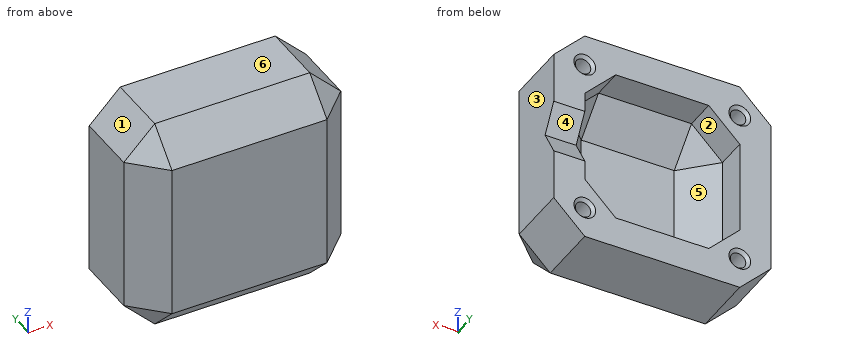
Autodesk Inventor part; units mm, degrees
ref_plane "YZ Plane" through (0, 0, 0) normal (1, 0, 0) x (0, 1, 0)
ref_plane "XZ Plane" through (0, 0, 0) normal (0, 1, 0) x (-1, 0, 0)
ref_plane "XY Plane" through (0, 0, 0) normal (0, 0, 1) x (1, 0, 0)
sketch "Sketch2" plane through (0, 0, 0) normal (0, 1, 0) x (-1, 0, 0)
  line L0 (25, -25) -> (-25, -25)
  line L1 (-25, -25) -> (-25, 25)
  line L2 (-25, 25) -> (25, 25)
  line L3 (25, 25) -> (25, -25)
  line L4 (25, -25) -> (-25, 25) construction
  line L5 (-25, -25) -> (25, 25) construction
  line L6 (35, 35) -> (-35, 35)
  line L7 (-35, 35) -> (-35, -35)
  line L8 (-35, -35) -> (35, -35)
  line L9 (35, -35) -> (35, 35)
  point P0 (0, 0)
  dimension "d0" = 50
  dimension "d1" = 10
  dimension "d19" = 50
extrude "Extrusion1" add sketch "Sketch2" along normal mid plane 30
sketch "Sketch3" plane through (0, -15, 0) normal (0, -1, 0) x (1, 0, 0)
  line L0 (35, -35) -> (35, 35)
  line L1 (35, 35) -> (-35, 35)
  line L2 (-35, 35) -> (-35, -35)
  line L3 (-35, -35) -> (35, -35)
  point P0 (0, 0)
extrude "Extrusion2" add sketch "Sketch3" against normal blind 10
chamfer "Chamfer1" distance 10 angle 45 16 edges at (35, 0, 35) (25, 5, 25) (-25, 5, 25) (-35, 0, 35) (-25, 5, -25) (25, 5, -25) (-35, 0, -35) (35, 0, -35) (0, -5, -25) (25, -5, 0) (0, -5, 25) (-25, -5, 0) (0, -15, -35) (35, -15, 0) (0, -15, 35) (-35, -15, 0)
sketch "Sketch4" plane through (35, -5, -25) normal (1, 0, 0) x (0, 0, -1)
  line L0 (0, 20) -> (0, 0) construction
  line L1 (-50, 20) -> (0, 20) construction
  line L2 (-16.3397, 30) -> (-16.3397, 20)
  line L3 (-16.3397, 20) -> (-25, 15)
  line L4 (-25, 15) -> (-33.6603, 20)
  line L5 (-33.6603, 20) -> (-33.6603, 30)
  line L6 (-33.6603, 30) -> (-25, 35)
  line L7 (-25, 35) -> (-16.3397, 30)
  point P0 (-25, 5)
  point P1 (-25, 25)
  dimension "d9" = 10
  dimension "d10" = 5
  dimension "d20" = 0
extrude "Extrusion3" cut sketch "Sketch4" against normal blind 10
sketch "Sketch5" plane through (0, 15, 0) normal (0, 1, 0) x (1, 0, 0)
  line L0 (-25, 25) -> (-25, 35) construction
  circle A0 centre (-25, 25) radius 2.5
  line L1 (25, 25) -> (35, 25) construction
  circle A1 centre (25, 25) radius 2.5
  line L2 (-25, -25) -> (-35, -25) construction
  circle A2 centre (-25, -25) radius 2.5
  line L3 (-25, -25) -> (25, -25) construction
  circle A3 centre (25, -25) radius 2.5
  point P0 (0, 0)
  dimension "d13" = 5
  dimension "d14" = 5
  dimension "d15" = 5
  dimension "d16" = 5
extrude "Extrusion4" cut sketch "Sketch5" against normal blind 10
chamfer "Chamfer2" distance 1 angle 45 4 edges at (-27.5, 15, 25) (-27.5, 15, -25) (22.5, 15, 25) (22.5, 15, -25)
properties part number "pokemon_ball_white"
Build history of the part. All positions in model axes, mm. Face numbers are marked on the shaded views. A direction names the side the tool comes from. Round coordinates to 2 decimals unless told otherwise and drop trailing zeros. Write each loop counter-clockwise with the first axis right and the second up, starting at its lowest first coordinate (ties: lowest second). Pieces come first, ordered by that corner, then holes. Notation, with made-up numbers: M 82,55.25 L 120,55.25 A16 ccw 120,67.25 Z; hole C 45.5,55.25 d8. An arc over 180 degrees is marked long. Answer as a JSON object with one key per item and string values. Group by question number.
(1) Which spindle directions (+Z, -Z, +X, -X, +Y, -Y) get a long thin tool onto all of the face, cutting with end or side? Do the marked faces 4, 5 and 6. Say none if no direction does.
(2) Drill centre lines: L1, parallel to Z at x = -8, y = 9; L2, parallel to Y at x = 10.5, z = -2; L3, parallel to X at y = 3.5, z = 31.5. Where is each one in solid material? Low to high.
(3) Cut at B-B (x = 19). Give the cut face in (y, z), and give its area (3 significant figures).
(4) Cut at D-D (z = -11). Give the cut face in (x, y), and give its area (3 significant figures).
(5) Mould opens along X. For the marked faces 1, 2 and 3 say: pulls with the +X half, pulls with the -X half, needs draft (parallel to the pull), parting line crosses it, or undercut.
(6) Cut at C-C (y = 8). Give the cut face in (x, z), and give its area (3 significant figures).
(7) Flat gauge pins, fed straight in: pin 1 (5.5 mm diameter, centred on x = 25, z = 25.5, fed in from +Y); pin 2 (4 mm diameter, centred on x = 24, z = -26, fed in from +Y); pin 3 (3 mm diameter, centred on x = 25, z = -25, fed in from +Y); pin 4 (5.5 mm diameter, centred on x = -26, z = 25.5, fed in from +Y). Where does each tip first touch, or does it go through?
(8) Cut at A-A (y = -4). Give the cut face in (x, z), and give its area (3 significant figures).
Responses:
{
 "1": {"face 4": "+X, +Y", "face 5": "+Y", "face 6": "+Z, +X, -X, +Y, -Y"},
 "2": {"L1": "z = -35 to -25, 25 to 35", "L2": "y = -15 to -5", "L3": "x = -28.5 to 28.5"},
 "3": {"outline": "M -15,-25 L -5,-35 L 15,-35 L 15,-21 L 5,-21 L -1,-15 L -1,15 L 5,21 L 15,21 L 15,35 L -5,35 L -15,25 Z", "area": "1,360 mm2"},
 "4": {"outline": "M -35,-5 L -25,-15 L 25,-15 L 35,-5 L 35,15 L 25,15 L 25,5 L 15,-5 L -15,-5 L -25,5 L -25,15 L -35,15 Z", "area": "1,100 mm2"},
 "5": {"face 1": "pulls with the -X half", "face 2": "undercut", "face 3": "pulls with the +X half"},
 "6": {"outline": "M -35,-25 L -25,-35 L 25,-35 L 35,-25 L 35,25 L 25,35 L -25,35 L -35,25 Z; hole C -25,-25 d5; hole C -25,25 d5; hole M -25,-15 L -15,-25 L 15,-25 L 25,-15 L 25,15 L 15,25 L -15,25 L -25,15 Z; hole C 25,-25 d5; hole C 25,25 d5", "area": "2,320 mm2"},
 "7": {"pin 1": "stops at y = 14.75", "pin 2": "stops at y = 14.91", "pin 3": "stops at y = 5", "pin 4": "stops at y = 15"},
 "8": {"outline": "M -35,-25 L -25,-35 L 25,-35 L 35,-25 L 35,25 L 25,35 L -25,35 L -35,25 Z; hole M -16,-15 L -15,-16 L 15,-16 L 16,-15 L 16,15 L 15,16 L -15,16 L -16,15 Z", "area": "3,680 mm2"}
}
